Design review of the part built by this model. Coordinates are the model's own, in mm. A direction names the side the tool comes from. Round coordinates to 2 decimals unless told otherwise and drop trailing zeros. Order: outer loops, then holes, each group sorted by start corner. A loop starts at its lowest first (then second) coordinate and runs counter-clockwise, first axis right, second up. Notation, with made-up numbers: M -0.5,-33 L 17.5,-33 A7 cw 17.5,-24 Z; hole C 9,47 d9. An arc over 180 degrees is marked long. Use a Markdown table: item, result. Add a question column.
(1) Take a section at C-C (y = 12.5). Write out the cut boundary in (x, z).
(2) For pin 1 (4.5 mm diameter, centred on x = 21.42, z = 32.7, fed in from +Y); pin 2 (3 mm diameter, centred on x = 10, z = 13, fed in from -Y); pin 3 (0.8 mm diameter, centred on x = 22, z = 33, fed in from +Y), all flat-tipped, find the tip position at first contact; note any pin that passes through.
(3) Machinability: for faces 1 (the face through (5.423, 7, 22)), 2 (the face through (1, 10.544, 33)), 3 (the face through (2, 4.044, 22)), which of the approach directions +Z, -Z, +X, -X, +Y, -Y give a long, thin tool a straight path to every point of the face, cutting with its end or side? Answer none if there is none.
(4) The part is to be moulded in two halves that separate along X. For faces 4 (the face through (12, 10, 0)), 5 (the face through (1, 10.544, 13)), 6 (the face through (-2.077, 9, 22)), 7 (the face through (17.423, 7, 22)), say which applies: released by +X, released by -X, zero draft, split by the parting line, or undercut.
(5) To check wall thickness, follow probe 1 along X at (y, z) = (11.5, 12.7); probe 2 along Z at (x, y) = (1.5, 13); probe 3 along X at (y, z) = (6, 12.5). State the ranges of each line that lie inside material, in increasing order. Write a range as from..to.
(6) Take a section at D-D (z = 17). Write out the cut boundary in (x, y), then the cut area to 4 significant figures.
(7) Take a section at A-A (y = 5.25). Write out the cut boundary in (x, z), then the cut area to 3 significant figures.
(8) Take a section at B-B (z = 32.7). Write out the cut boundary in (x, y).
```python
from build123d import *

# Parameters (mm, degrees)
EXTRUDE_1_DEPTH     = 45.4
HOLE_WIZARD_2_D     = 2.8
HOLE_WIZARD_2_DEPTH = 3.5


with BuildPart() as part:
    # 草图1 → 凸台-拉伸1 (new body)
    with BuildSketch(Plane.XY):
        Polygon((-1.576923077, 14.043956044), (24.423076923, 14.043956044), (24.923076923, 13.543956044), (24.923076923, 4.543956044), (24.423076923, 4.043956044), (17.423076923, 4.043956044), (17.423076923, 9.043956044), (5.423076923, 9.043956044), (5.423076923, 4.043956044), (-1.576923077, 4.043956044), (-2.076923077, 4.543956044), (-2.076923077, 13.543956044), align=None)
    extrude(amount=EXTRUDE_1_DEPTH)

    # 孔2
    with Locations(Plane(origin=(21.423076923, 14.043956044, 32.7), x_dir=(0, 0, 1), z_dir=(0, 1, 0))):
        with Locations((0, 0), (-20, 0), (-20, -20), (0, -20)):
            Hole(HOLE_WIZARD_2_D / 2, depth=HOLE_WIZARD_2_DEPTH)


solid = part.part
```
Verdict:
| question | item | result |
|---|---|---|
| 1 | outline | M -2.08,0 L 24.92,0 L 24.92,45.4 L -2.08,45.4 Z; hole C 1.42,12.7 d2.8; hole C 1.42,32.7 d2.8; hole C 21.42,12.7 d2.8; hole C 21.42,32.7 d2.8 |
| 2 | pin 1 | stops at y = 14.04 |
| 2 | pin 2 | stops at y = 9.04 |
| 2 | pin 3 | stops at y = 10.54 |
| 3 | face 1 | +Z, -Z, -Y |
| 3 | face 2 | +Y |
| 3 | face 3 | +Z, -Z, +X, -X, -Y |
| 4 | face 4 | zero draft |
| 4 | face 5 | undercut |
| 4 | face 6 | released by -X |
| 4 | face 7 | undercut |
| 5 | probe 1 | x = -2.08..0.02, 2.82..20.02, 22.82..24.92 |
| 5 | probe 2 | z = 0..11.3, 14.1..31.3, 34.1..45.4 |
| 5 | probe 3 | x = -2.08..5.42, 17.42..24.92 |
| 6 | outline | M -2.08,4.54 L -1.58,4.04 L 5.42,4.04 L 5.42,9.04 L 17.42,9.04 L 17.42,4.04 L 24.42,4.04 L 24.92,4.54 L 24.92,13.54 L 24.42,14.04 L -1.58,14.04 L -2.08,13.54 Z |
| 6 | area | 209.5 mm^2 |
| 7 | outline | M -2.08,0 L 5.42,0 L 5.42,45.4 L -2.08,45.4 Z; M 17.42,0 L 24.92,0 L 24.92,45.4 L 17.42,45.4 Z |
| 7 | area | 681 mm^2 |
| 8 | outline | M -2.08,4.54 L -1.58,4.04 L 5.42,4.04 L 5.42,9.04 L 17.42,9.04 L 17.42,4.04 L 24.42,4.04 L 24.92,4.54 L 24.92,13.54 L 24.42,14.04 L 22.82,14.04 L 22.82,10.54 L 20.02,10.54 L 20.02,14.04 L 2.82,14.04 L 2.82,10.54 L 0.02,10.54 L 0.02,14.04 L -1.58,14.04 L -2.08,13.54 Z |
